Here's how the part is built. I have some questions about the finished solid (model axes, mm). Face numbers are marked on the shaded views. A direction names the side the tool comes from. Round coordinates to 2 decimals unless told otherwise and drop trailing zeros. Loops run counter-clockwise (first coordinate to the right, second up) from the corner with the lowest first, then second, coordinate; pieces in that order, holes last. Notation, with made-up numbers: (-22, 42.5) -> (15, 42.5) arc R18 ccw to (15, 61.5) -> close; hole circle Ø9 at (64, 51). An arc over 180 degrees is marked (long way). Use one line per item in the form item = value. Start each with the question number.
Item 1: If we section it at C-C (y = 27.5): Write out the boundary of the cut face in (x, z), then the cut area to 3 significant figures.
Item 2: For the marked faces 1, 2 and 3, which set-ups out of +Z, -Z, +X, -X, +Y, -Y let a thin tool reach every point of the face, with its end or its side?
Item 3: I'm going to push flat-ended pins straight in: pin 1 Ø3 at (x, z) = (4.5, -1.5) entering from +Y; pin 2 Ø2.5 at (y, z) = (2.8, 0) entering from +X; pin 3 Ø2.5 at (y, z) = (4.5, 3.25) entering from +X. Where does each tip first touch, or does it pass through?
Item 4: If I drill on L1, parallel to Y at x = 1.5, z = 0; L2, parallel to Z at x = 6.5, y = 4.5; L3, parallel to Z at x = 3.5, y = 5.3, over which ranges is the centre line in solid material (lowest first)? Write a range as [from, to].
Item 5: If we section it at A-A (x = 1.5): Write out the boundary of the cut face in (y, z).
Item 6: If we section it at D-D (y = 9): Write out the boundary of the cut face in (x, z).
Item 7: If we section it at B-B (z = -3.75): Write out the boundary of the cut face in (x, y), then the cut area to 3 significant figures.
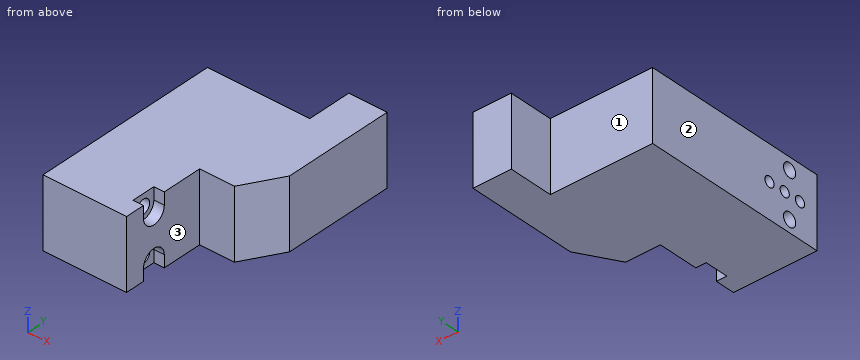
Autodesk Inventor part; units mm, degrees
ref_plane "YZ Plane" through (0, 0, 0) normal (1, 0, 0) x (0, 1, 0)
ref_plane "XZ Plane" through (0, 0, 0) normal (0, 1, 0) x (-1, 0, 0)
ref_plane "XY Plane" through (0, 0, 0) normal (0, 0, 1) x (1, 0, 0)
sketch "Skizze1" plane through (0, 0, 0) normal (0, 0, 1) x (1, 0, 0)
  line L0 (0, 40.08) -> (0, -6.68)
  line L1 (-4.04, 0) -> (24.24, 0)
  line L2 (0, 0) -> (12, 0)
  line L3 (12, 0) -> (12, 12)
  line L4 (14.7, 27) -> (0, 27)
  line L5 (0, 27) -> (0, 0)
  line L6 (14.7, 27) -> (14.7, 33.4)
  line L7 (14.7, 33.4) -> (20.2, 33.4)
  line L8 (20.2, 33.4) -> (20.2, 17.4)
  line L9 (20.2, 17.4) -> (17, 12)
  line L10 (17, 12) -> (12, 12)
  dimension "d0" = 5.5
  dimension "d1" = 14.7
  dimension "d3" = 12
  dimension "d4" = 27
  dimension "d5" = 12
  dimension "d6" = 5
  dimension "d7" = 6.4
  dimension "d8" = 16
extrude "Extrusion1" add sketch "Skizze1" along normal mid plane 10
hole "Bohrung1" at (12, 4.5, 3.25) direction (-1, 0, 0) diameter 2 end up to surface counterbore diameter 3.4 counterbore depth 1.5
sketch "Skizze2" plane through (12, 0, -5) normal (1, 0, 0) x (0, 0, -1)
  circle A0 centre (-8.25, 4.5) radius 1.7
  line L0 (-10, 0) -> (-10, 27)
  line L1 (-10, 2.8) -> (-8.25, 2.8)
  line L2 (-8.25, 2.8) -> (-8.25, 6.2)
  line L3 (-8.25, 6.2) -> (-10, 6.2)
  line L4 (-10, 6.2) -> (-10, 2.8)
  point P0 (-10, 5.3874)
  point P1 (-10, 3.6126)
extrude "Extrusion2" cut sketch "Skizze2" against normal up to surface (1.5 mm away) contours L2 A0 | A0 L1 L0 L3 picked at (-8.7614, 4.0923)
mirror "Spiegeln1" about plane through (0, 0, 0) normal (0, 0, 1) of "Bohrung1", "Extrusion2"
sketch "Skizze3" plane through (0, 0, 5) normal (-1, 0, 0) x (0, 0, 1)
  line L0 (0, 0) -> (0, 27)
  line L1 (0, 0) -> (-10, 0)
  circle A0 centre (-1.75, 4.5) radius 1
  point P0 (-5, 2.8)
  point P1 (-5, 5.3)
  point P2 (-5, 7.8)
  dimension "d22" = 2.5
  dimension "d23" = 2.5
  dimension "d24" = 2.8
  dimension "d25" = 7.8
  dimension "d26" = 5
  dimension "d27" = 5.3
  dimension "d35" = 0.8
hole "Bohrung2" at (0, 2.8, 0) at (0, 5.3, 0) at (0, 7.8, 0) direction (1, 0, 0) diameter 1.5 depth 8 tip angle 118
properties part number "Valve_Outside"
Values found:
q1.outline = (14.7, -5) -> (20.2, -5) -> (20.2, 5) -> (14.7, 5) -> close
q1.area = 55.0 mm2
q2.face_1 = +Z, -Z, -X, +Y
q2.face_2 = +Z, -Z, -X, +Y, -Y
q2.face_3 = +Z, -Z, +X, -Y
q3.pin_1 = 27
q3.pin_2 = 12
q3.pin_3 = 10.5
q4.L1 = [0, 2.05], [3.55, 4.55], [6.05, 7.05], [8.55, 27]
q4.L2 = [-5, -4.25], [-2.25, 2.25], [4.25, 5]
q4.L3 = [-5, -3.85], [-2.65, -0.75], [0.75, 2.65], [3.85, 5]
q5.outline = (0, -5) -> (27, -5) -> (27, 5) -> (0, 5) -> close; hole circle Ø1.5 at (2.8, 0); hole circle Ø2 at (4.5, -3.25); hole circle Ø2 at (4.5, 3.25); hole circle Ø1.5 at (5.3, 0); hole circle Ø1.5 at (7.8, 0)
q6.outline = (0, -5) -> (12, -5) -> (12, 5) -> (0, 5) -> close
q7.outline = (0, 0) -> (12, 0) -> (12, 2.8) -> (10.5, 2.8) -> (10.5, 3.63) -> (0, 3.63) -> close; (0, 5.37) -> (10.5, 5.37) -> (10.5, 6.2) -> (12, 6.2) -> (12, 12) -> (17, 12) -> (20.2, 17.4) -> (20.2, 33.4) -> (14.7, 33.4) -> (14.7, 27) -> (0, 27) -> close
q7.area = 450 mm2
